```python
from build123d import *

# Parameters (mm, degrees)
F0_R     = 2.54
F1_DEPTH = 6.35
F0_R_2   = 63.5
F2_DEPTH = 3.81
F3_R     = 1.905
F4_DEPTH = 40.64
F5_R     = 1.5875
F6_DEPTH = 25.4


with BuildPart() as f1:
    # F0 (on Top) → F1 (new body)
    with BuildSketch(Plane.XY):
        Circle(F0_R)
    extrude(amount=F1_DEPTH)

    # F0 (on Top) → F2 (join)
    with BuildSketch(Plane.XY):
        Circle(F0_R_2)
        Circle(F0_R, mode=Mode.SUBTRACT)
    extrude(amount=F2_DEPTH)

    # F3 (on face) → F4 (cut)
    with BuildSketch(Plane.XY.offset(6.35)):
        Circle(F3_R)
    extrude(amount=-F4_DEPTH, mode=Mode.SUBTRACT)

    # F5 (on face) → F6 (cut)
    with BuildSketch(Plane(origin=(0, 0, 0), x_dir=(1, 0, 0), z_dir=(0, 0, -1))):
        with Locations((44.45, 0)):
            Circle(F5_R)
        with Locations((-44.45, 0)):
            Circle(F5_R)
    extrude(amount=-F6_DEPTH, mode=Mode.SUBTRACT)


solid = f1.part
```
Here's how the part is built. I have some questions about the finished solid (model axes, mm). A direction names the side the tool comes from. Coordinates: 2 decimals unless noted, no trailing zeros. Order: outer loops, then holes, each group sorted by start corner. A loop starts at its lowest first (then second) coordinate and runs counter-clockwise, first axis right, second up. Notation, with made-up numbers: M -11.75,57.5 L 31.25,57.5 A15 ccw 31.25,74.5 Z; hole C 41.5,32 d11. An arc over 180 degrees is marked long. Answer as a JSON object with one key per item and string values. Group by question number.
(1) Suppose I cut it at A-A, the plane x = 0. Please give me the cut outline in (y, z) (3 decimals).
(2) Suppose I cut it at D-D, the plane y = 49. Please give me the cut outline in (x, z).
(3) I need wall thicknesses on probe 1 along Y at (x, z) = (0, 1.5) (3 decimals); probe 2 along Z at (x, y) = (-19.5, 40); probe 3 along Y at (x, z) = (54, 1.5). Which ranges of each line are inside material? Lowest first, please.
(4) Suppose I cut it at C-C, the plane x = -44.45. Please give me the cut outline in (y, z).
(5) For pin 1 (3.5 mm diameter, centred on x = 0, y = 0, fed in from +Z); pin 2 (1.5 mm diameter, centred on x = -6, z = 2, fed in from -Y); pin 3 (1 mm diameter, centred on x = 42, z = 3, fed in from -Y); pin 4 (5 mm diameter, centred on x = 49.5, y = -32, fed in from +Z), each with a flat end and sliding along its axis, tell me the tip position at first contact or that it passes through.
(6) Which directions (+Z, -Z, +X, -X, +Y, -Y) give clear straight access to the entire face, cutting with the end or side of a thin tool? Please do faces 1 (the face through (-0.33, 2.52, 5.06)), 2 (the face through (-0.41, -1.86, 3.22)).
(7) Suppose I cut it at B-B, the plane y = 0. State how many separate pieces and enclosed holes the cut face has, then the cut area to 3 significant figures.
Values found:
{
 "1": {"outline": "M -63.5,0 L -1.905,0 L -1.905,6.35 L -2.54,6.35 L -2.54,3.81 L -63.5,3.81 Z; M 1.905,0 L 63.5,0 L 63.5,3.81 L 2.54,3.81 L 2.54,6.35 L 1.905,6.35 Z"},
 "2": {"outline": "M -40.39,0 L 40.39,0 L 40.39,3.81 L -40.39,3.81 Z"},
 "3": {"probe 1": "y = -63.5 to -1.905, 1.905 to 63.5", "probe 2": "z = 0 to 3.81", "probe 3": "y = -33.41 to 33.41"},
 "4": {"outline": "M -45.35,0 L -1.59,0 L -1.59,3.81 L -45.35,3.81 Z; M 1.59,0 L 45.35,0 L 45.35,3.81 L 1.59,3.81 Z"},
 "5": {"pin 1": "passes through", "pin 2": "stops at y = -63.28", "pin 3": "stops at y = -48.06", "pin 4": "stops at z = 3.81"},
 "6": {"face 1": "+Z", "face 2": "+Z, -Z"},
 "7": {"separate pieces": "4", "enclosed holes": "0", "area": "448 mm^2"}
}
